```python
from build123d import *

# Parameters (mm, degrees)
SKETCH1_W           = 93.85
SKETCH1_H           = 54.4
SKETCH1_W_2         = 89.85
SKETCH1_H_2         = 50.4
SKETCH1_W_3         = 8.5
SKETCH1_W_4         = 72.85
BOSS_EXTRUDE1_DEPTH = 2
SKETCH2_W           = 93.85
SKETCH2_H           = 54.4
SKETCH2_W_2         = 86
SKETCH2_H_2         = 50
BOSS_EXTRUDE2_DEPTH = 10
SKETCH3_W           = 8.45
SKETCH3_H           = 50
SKETCH3_W_2         = 69.9
SKETCH3_H_2         = 2
SKETCH3_W_3         = 7.65
BOSS_EXTRUDE3_DEPTH = 3
SKETCH5_W           = 10
SKETCH5_H           = 6.29
SKETCH5_W_2         = 11.1
SKETCH5_H_2         = 6.9
CUT_EXTRUDE1_DEPTH  = 5.85
SKETCH6_W           = 86
SKETCH6_H           = 50
BOSS_EXTRUDE4_DEPTH = 2.6
SKETCH8_W           = 86
SKETCH8_H           = 7.4
CUT_EXTRUDE2_DEPTH  = 2.4
SKETCH9_W           = 7.65
SKETCH9_H           = 52.4
SKETCH9_W_2         = 8.45
BOSS_EXTRUDE5_DEPTH = 0.95
SKETCH13_W          = 52.4
SKETCH13_H          = 6.45
CUT_EXTRUDE4_DEPTH  = 3
SKETCH14_W          = 52.4
SKETCH14_H          = 6.45
CUT_EXTRUDE5_DEPTH  = 1.5
FILLET1_R           = 2
FILLET2_R           = 1


with BuildPart() as part:
    # Sketch1 → Boss-Extrude1 (new body)
    # profile 1 of 4: a face of its own
    with BuildSketch(Plane(origin=(0, 0, 0), x_dir=(1, 0, 0), z_dir=(0, 1, 0))):
        with Locations((44.925, 25.2)):
            Rectangle(SKETCH1_W, SKETCH1_H)
        with Locations((44.925, 25.2)):
            Rectangle(SKETCH1_W_2, SKETCH1_H_2, mode=Mode.SUBTRACT)
    # profile 2 of 4: a face of its own
    with BuildSketch(Plane(origin=(0, 0, 0), x_dir=(1, 0, 0), z_dir=(0, 1, 0))):
        with Locations((4.25, 25.2)):
            Rectangle(SKETCH1_W_3, SKETCH1_H_2)
    # profile 3 of 4: a face of its own
    with BuildSketch(Plane(origin=(0, 0, 0), x_dir=(1, 0, 0), z_dir=(0, 1, 0))):
        with Locations((44.925, 25.2)):
            Rectangle(SKETCH1_W_4, SKETCH1_H_2)
    # profile 4 of 4: a face of its own
    with BuildSketch(Plane(origin=(0, 0, 0), x_dir=(1, 0, 0), z_dir=(0, 1, 0))):
        with Locations((85.6, 25.2)):
            Rectangle(SKETCH1_W_3, SKETCH1_H_2)
    extrude(amount=BOSS_EXTRUDE1_DEPTH)

    # Sketch2 → Boss-Extrude2 (add)
    with BuildSketch(Plane(origin=(0, 2, 0), x_dir=(1, 0, 0), z_dir=(0, 1, 0))):
        with Locations((44.925, 25.2)):
            Rectangle(SKETCH2_W, SKETCH2_H)
        with Locations((43, 25)):
            Rectangle(SKETCH2_W_2, SKETCH2_H_2, mode=Mode.SUBTRACT)
    extrude(amount=BOSS_EXTRUDE2_DEPTH)

    # Sketch3 → Boss-Extrude3 (add)
    with BuildSketch(Plane(origin=(0, 12, 0), x_dir=(1, 0, 0), z_dir=(0, 1, 0))):
        with Locations((4.225, 25)):
            Rectangle(SKETCH3_W, SKETCH3_H)
        Polygon((8.45, 52.4), (-2, 52.4), (-2, -2), (8.45, -2), (8.45, 0), (0, 0), (0, 50), (8.45, 50), align=None)
        with Locations((43.4, -1)):
            Rectangle(SKETCH3_W_2, SKETCH3_H_2)
        with Locations((82.175, 25)):
            Rectangle(SKETCH3_W_3, SKETCH3_H)
        Polygon((91.85, 52.4), (78.35, 52.4), (78.35, 50), (86, 50), (86, 0), (78.35, 0), (78.35, -2), (91.85, -2), align=None)
    extrude(amount=BOSS_EXTRUDE3_DEPTH)

    # Sketch5 → Cut-Extrude1 (cut)
    with BuildSketch(Plane.ZY.offset(-86)):
        with Locations((-33.95, 8.845)):
            Rectangle(SKETCH5_W, SKETCH5_H)
        with Locations((-15, 8.54)):
            Rectangle(SKETCH5_W_2, SKETCH5_H_2)
    extrude(amount=-CUT_EXTRUDE1_DEPTH, mode=Mode.SUBTRACT)

    # Sketch6 → Boss-Extrude4 (add)
    with BuildSketch(Plane(origin=(0, 2, 0), x_dir=(1, 0, 0), z_dir=(0, 1, 0))):
        with Locations((43, 25)):
            Rectangle(SKETCH6_W, SKETCH6_H)
    extrude(amount=BOSS_EXTRUDE4_DEPTH)

    # Sketch8 → Cut-Extrude2 (cut)
    with BuildSketch(Plane.XY.offset(-50)):
        with Locations((43, 8.3)):
            Rectangle(SKETCH8_W, SKETCH8_H)
    extrude(amount=-CUT_EXTRUDE2_DEPTH, mode=Mode.SUBTRACT)

    # Sketch9 → Boss-Extrude5 (add)
    with BuildSketch(Plane.XZ.offset(-12)):
        with Locations((82.175, -26.2)):
            Rectangle(SKETCH9_W, SKETCH9_H)
        with Locations((4.225, -26.2)):
            Rectangle(SKETCH9_W_2, SKETCH9_H)
    extrude(amount=BOSS_EXTRUDE5_DEPTH)

    # Sketch13 → Cut-Extrude4 (cut)
    with BuildSketch(Plane.ZY.offset(-86)):
        with Locations((-26.2, 7.825)):
            Rectangle(SKETCH13_W, SKETCH13_H)
    extrude(amount=-CUT_EXTRUDE4_DEPTH, mode=Mode.SUBTRACT)

    # Sketch14 → Cut-Extrude5 (cut)
    with BuildSketch(Plane.ZY.offset(-89)):
        with Locations((-26.2, 7.825)):
            Rectangle(SKETCH14_W, SKETCH14_H)
    extrude(amount=-CUT_EXTRUDE5_DEPTH, mode=Mode.SUBTRACT)

    # Fillet1
    fillet1_edges = [part.edges().sort_by_distance(p)[0] for p in [
        (0, 7.825, 0),
        (90.5, 7.825, 0),
    ]]
    fillet(fillet1_edges, radius=FILLET1_R)

    # Fillet2
    fillet2_edges = [part.edges().sort_by_distance(p)[0] for p in [
        (91.85, 7.5, 2),
        (-2, 7.5, 2),
        (-2, 7.5, -52.4),
        (91.85, 7.5, -52.4),
    ]]
    fillet(fillet2_edges, radius=FILLET2_R)


solid = part.part
```
Could you check a few things on this model? Use its own coordinates, in mm. A direction names the side the tool comes from. Round coordinates to 2 decimals unless told otherwise and drop trailing zeros. Loops run counter-clockwise (first coordinate to the right, second up) from the corner with the lowest first, then second, coordinate; pieces in that order, holes last.
Q1. I want a section at B-B (y = 8.5). Write out the boundary of the cut face in (x, z), and give its area (3 significant figures).
Q2. I want a section at A-A (z = -36). Write out the boundary of the cut face in (x, y), and give its area (3 significant figures).
Q3. Thinking about a two-plate mould opening in Z: for faces 1 (the flat face through (44, 4, -52.4)), 2 (the flat face through (91, 10, -38.95)), 3 (the flat face through (44, 0, -26)), which applies, pulls with the +Z half, pulls with the -Z half, needs draft (parallel to the pull), parting line crosses it, or undercut?
Q4. For P1, Ø4.5, axis at x = 88.5, z = -13, coming from the -Y side; P2, Ø0.8, axis at y = 11.5, z = -15, coming from the +X side; P3, Ø2, axis at x = 42, z = -11.5, coming from the +Y side, each with a flat end and sliding along its axis, tell me the tip position at first contact or that it passes through.
Q5. On a 3-axis mill with a long thin cutter (end or side, diameter ignored), from which of +Z, -Z, +X, -X, +Y, -Y can I reach the whole of each face in a straight line? I mean faces 4 (the flat face through (-2, 7, -26)), 5 (the flat face through (91, 10, -28.95)), 6 (the cylindrical face through (89.93, 7.87, -0.6)), 7 (the flat face through (8.45, 13, -27)), 8 (the flat face through (91.85, 7, -25)). Say none if no direction works.
Q6. I want a section at C-C (x = 82.5). Write out the boundary of the cut face in (y, z).
Q7. I want a section at D-D (z = -15). Write out the boundary of the cut face in (x, y).
Q8. Please list where these lines run through material, in increasing order: L1, parallel to X at y = 8.75, z = -5; L2, parallel to X at y = 14.5, z = -2; L3, parallel to Y at x = 5.5, z = -47.
Answer below:
1. outline: (-2, -51.4) arc R1 ccw to (-1, -52.4) - (0, -52.4) - (0, -2) arc R2 cw to (2, 0) - (88.5, 0) arc R2 cw to (90.5, -2) - (90.5, -9.45) - (91.85, -9.45) - (91.85, 1) arc R1 ccw to (90.85, 2) - (-1, 2) arc R1 ccw to (-2, 1) - close; (90.5, -52.4) - (90.85, -52.4) arc R1 ccw to (91.85, -51.4) - (91.85, -38.95) - (90.5, -38.95) - close; (90.5, -28.95) - (91.85, -28.95) - (91.85, -20.55) - (90.5, -20.55) - close
1. area: 336 mm2
2. outline: (-2, 0) - (91.85, 0) - (91.85, 5.7) - (90.5, 5.7) - (90.5, 4.6) - (0, 4.6) - (0, 11.05) - (8.45, 11.05) - (8.45, 15) - (-2, 15) - close; (78.35, 11.05) - (86, 11.05) - (86, 11.99) - (91.85, 11.99) - (91.85, 15) - (78.35, 15) - close
2. area: 535 mm2
3. face 1: pulls with the -Z half
3. face 2: undercut
3. face 3: needs draft
4. P1: stops at y = 0
4. P2: stops at x = 86
4. P3: stops at y = 4.6
5. face 4: +Z, -Z, -X, +Y, -Y
5. face 5: +X
5. face 6: -Z
5. face 7: -Z, +Y
5. face 8: +Z, -Z, +X, +Y, -Y
6. outline: (0, -52.4) - (4.6, -52.4) - (4.6, 0) - (11.05, 0) - (11.05, -52.4) - (15, -52.4) - (15, 2) - (0, 2) - close
7. outline: (-2, 0) - (91.85, 0) - (91.85, 5.09) - (90.5, 5.09) - (90.5, 4.6) - (0, 4.6) - (0, 11.05) - (8.45, 11.05) - (8.45, 15) - (-2, 15) - close; (78.35, 11.05) - (86, 11.05) - (86, 11.99) - (91.85, 11.99) - (91.85, 15) - (78.35, 15) - close
8. L1: x = -2 to 0, 90.5 to 91.85
8. L2: x = -2 to 8.45, 78.35 to 91.85
8. L3: y = 0 to 4.6, 11.05 to 15
